Solid Edge part; units mm, degrees
sketch "Sketch1" plane through (0, 0, 0) normal (0, 0, 1) x (1, 0, 0)
  line L0 (-54.5, -37) -> (54.5, -37)
  line L1 (54.5, -37) -> (54.5, 37)
  line L2 (54.5, 37) -> (-54.5, 37)
  line L3 (-54.5, 37) -> (-54.5, -37)
extrude "Protrusion1" add sketch "Sketch1" along normal blind 2
sketch "Sketch2" plane through (0, 0, 2) normal (0, 0, 1) x (1, 0, 0)
  line L0 (-54.5, 37) -> (54.5, 37)
  line L1 (54.5, 37) -> (54.5, -37)
  line L2 (54.5, -37) -> (-54.5, -37)
  line L3 (-54.5, -37) -> (-54.5, 37)
  line L4 (-53.5, 36) -> (-53.5, -36)
  line L5 (-53.5, -36) -> (53.5, -36)
  line L6 (53.5, -36) -> (53.5, 36)
  line L7 (53.5, 36) -> (-53.5, 36)
extrude "ExtrudedProtrusion_3" add sketch "Sketch2" along normal blind 3.5
sketch "Sketch3" plane through (0, 0, 2) normal (0, 0, 1) x (1, 0, 0)
  circle A0 centre (-43.5, 25.5) radius 2.845
  circle A1 centre (-43.5, -20.5) radius 2.845
  circle A2 centre (42.5, 25.5) radius 2.845
  circle A3 centre (42.5, -20.5) radius 2.845
extrude "ExtrudedProtrusion_4" add sketch "Sketch3" along normal blind 11.5
sketch "Sketch4" plane through (-42.5, 25.5, 13.5) normal (0, 0, 1) x (1, 0, 0)
  circle A0 centre (-1, 0) radius 1.5
  circle A1 centre (85, 0) radius 1.5
  circle A2 centre (85, -46) radius 1.5
  circle A3 centre (-1, -46) radius 1.5
extrude "ExtrudedCutout_1" cut sketch "Sketch4" against normal blind 4.7
sketch "Sketch5" plane through (0, 0, 2) normal (0, 0, 1) x (1, 0, 0)
  line L0 (-0.5627, 17.794) -> (-0.5627, -2.206)
  line L1 (-0.5627, -2.206) -> (-41.0627, -2.206)
  line L2 (-41.0627, -2.206) -> (-41.0627, -22.206)
  line L3 (-41.0627, -22.206) -> (38.9373, -22.206)
  line L4 (38.9373, -22.206) -> (38.9373, 17.794)
  line L5 (38.9373, 17.794) -> (-0.5627, 17.794)
extrude "Cutout1" cut sketch "Sketch5" against normal through all
Part model, mm, in its own coordinate system. A direction names the side the tool comes from. Round coordinates to 2 decimals unless told otherwise and drop trailing zeros. Order: outer loops, then holes, each group sorted by start corner. A loop starts at its lowest first (then second) coordinate and runs counter-clockwise, first axis right, second up. Notation, with made-up numbers: M 20,7.25 L 75,7.25 A26 cw 75,30.25 Z; hole C 78.5,-36.5 d7. An arc over 180 degrees is marked long. Answer in a Markdown table with one row per item. Add a question column.
Q1. Cut at A-A on y = 5.5. Give the cut face in (x, z), and give its area (3 significant figures).
Q2. Mould opens along X. For faces 1 (the face through (-54.5, 1, 3)), 2 (the face through (-42, -22, 13.5)), 3 (the face through (-45, -20.43, 11.18)) say: +X half, -X half, draft (parallel to the pull), parting line (faces both ways), or undercut.
Q3. Pin check, flat tips, straight feed: pin 1 (2 mm diameter, centred on x = -33, y = 13, fed in from +Z); pin 2 (4 mm diameter, centred on y = -17, z = 11, fed in from +X); pin 3 (1.5 mm diameter, centred on x = 42.5, y = 25, fed in from +Z). Stop position of each tip, or through.
Q4. 3-axis set-ups, long thin cutter, end or side, ignore diameter. For faces 4 (the face through (42.13, 22.68, 7.67)), 5 (the face through (-2, -22.206, 1)), 6 (the face through (1, 37, 3)): which of +Z, -Z, +X, -X, +Y, -Y reach the whole face in a straight line?
Q5. Cut at C-C on x = 37. Give the cut face in (y, z).
Q6. Cut at D-D on y = -20.5. Give the cut face in (x, z) (3 decimals), and give its area (3 significant figures).
Q7. Wall check: L1, parallel to Y at x = 42.5, z = 10.9 (3 decimals); L2, parallel to X at y = -5, z = 5; L3, parallel to Y at x = -28, z = 4. Give the ranges that are in metal, low to high. Write a range as from..to.
Q8. Cut at B-B on z = 10. Give the cut face in (x, y) (3 decimals), and give its area (3 significant figures).
Established:
| question | item | result |
|---|---|---|
| 1 | outline | M -54.5,0 L -0.56,0 L -0.56,2 L -53.5,2 L -53.5,5.5 L -54.5,5.5 Z; M 38.94,0 L 54.5,0 L 54.5,5.5 L 53.5,5.5 L 53.5,2 L 38.94,2 Z |
| 1 | area | 146 mm2 |
| 2 | face 1 | -X half |
| 2 | face 2 | draft |
| 2 | face 3 | undercut |
| 3 | pin 1 | stops at z = 2 |
| 3 | pin 2 | stops at x = 44.92 |
| 3 | pin 3 | stops at z = 8.8 |
| 4 | face 4 | +Z |
| 4 | face 5 | +Z, -Z |
| 4 | face 6 | +Z, -Z, +X, -X, +Y |
| 5 | outline | M -37,0 L -22.21,0 L -22.21,2 L -36,2 L -36,5.5 L -37,5.5 Z; M 17.79,0 L 37,0 L 37,5.5 L 36,5.5 L 36,2 L 17.79,2 Z |
| 6 | outline | M -54.5,0 L -41.063,0 L -41.063,2 L -40.655,2 L -40.655,13.5 L -42,13.5 L -42,8.8 L -45,8.8 L -45,13.5 L -46.345,13.5 L -46.345,2 L -53.5,2 L -53.5,5.5 L -54.5,5.5 Z; M 38.937,0 L 54.5,0 L 54.5,5.5 L 53.5,5.5 L 53.5,2 L 45.345,2 L 45.345,13.5 L 44,13.5 L 44,8.8 L 41,8.8 L 41,13.5 L 39.655,13.5 L 39.655,2 L 38.937,2 Z |
| 6 | area | 168 mm2 |
| 7 | L1 | y = -23.345..-22, -19..-17.655, 22.655..24, 27..28.345 |
| 7 | L2 | x = -54.5..-53.5, 53.5..54.5 |
| 7 | L3 | y = -37..-36, 36..37 |
| 8 | outline | C -43.5,-20.5 d5.69; C -43.5,25.5 d5.69; C 42.5,-20.5 d5.69; C 42.5,25.5 d5.69; hole C -43.5,-20.5 d3; hole C -43.5,25.5 d3; hole C 42.5,-20.5 d3; hole C 42.5,25.5 d3 |
| 8 | area | 73.4 mm2 |
